Could you check a few things on this drawing? It's one solid part, dimensions in mm from its lowest x, y, z. Give positions to 0.01 mm unless a question says otherwise; leave off trailing zeros. Write each loop counter-clockwise with the first axis right and the second up, starting at its lowest first coordinate (ties: lowest second). Pieces come first, ordered by that corner, then holes. Notation, with made-up numbers: (-3.75, 81.5) -> (8.25, 81.5) arc R19 cw to (8.25, 97.5) -> close; hole circle Ø7 at (-36.5, 77). An arc over 180 degrees is marked (long way). Answer as CSV lines item,"result". Start each with the question number.
1. If we section it at B-B on x = 8.5: Write out the boundary of the cut face in (y, z), plus the area to 3 significant figures.
2. I need wall thicknesses on line 1 (X direction, y = 3.8, z = 31); line 2 (Z direction, x = 8, y = 3.4); line 3 (Z direction, x = 55, y = 3.1) (1 decimal). Which ranges of each line are inside material? Lowest first, please. Write a range as [from, to].
3. If we section it at C-C on z = 13: Write out the boundary of the cut face in (x, y), plus the area to 3 significant figures.
4. I'm going to push flat-ended pins straight in: P1, Ø2, axis at x = 19, z = 51.5, coming from the -Y side; P2, Ø1.4, axis at y = 3, z = 12, coming from the -X side; P3, Ø1.4, axis at x = 70, y = 2, coming from the -Z side. Where does each tip first touch, or does it pass through?
5. If we section it at A-A on y = 3.05: Write out the boundary of the cut face in (x, z), plus the area to 3 significant figures.
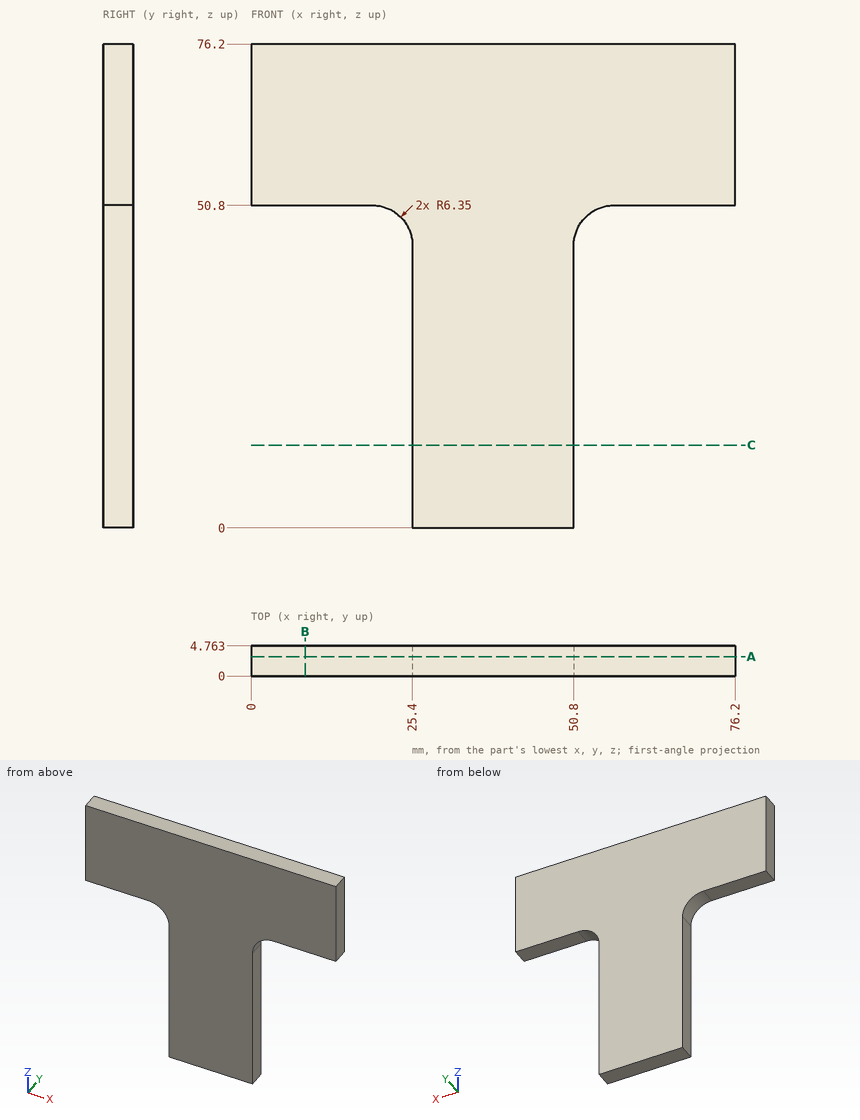
Computed values:
1,outline,"(0, 50.8) -> (4.76, 50.8) -> (4.76, 76.2) -> (0, 76.2) -> close"
1,area,"121 mm2"
2,line 1,"x = [25.4, 50.8]"
2,line 2,"z = [50.8, 76.2]"
2,line 3,"z = [50.4, 76.2]"
3,outline,"(25.4, 0) -> (50.8, 0) -> (50.8, 4.76) -> (25.4, 4.76) -> close"
3,area,"121 mm2"
4,P1,"stops at y = 0"
4,P2,"stops at x = 25.4"
4,P3,"stops at z = 50.8"
5,outline,"(0, 50.8) -> (19.05, 50.8) arc R6.35 cw to (25.4, 44.45) -> (25.4, 0) -> (50.8, 0) -> (50.8, 44.45) arc R6.35 cw to (57.15, 50.8) -> (76.2, 50.8) -> (76.2, 76.2) -> (0, 76.2) -> close"
5,area,"3,240 mm2"
